Build history of the part. All positions in model axes, mm. A direction names the side the tool comes from. Coordinates: 2 decimals unless noted, no trailing zeros. Loops run counter-clockwise (first coordinate to the right, second up) from the corner with the lowest first, then second, coordinate; pieces in that order, holes last.
Item 1: Mould opens along Z. For faces 6 (the face through (9, 27, 332)), 7 (the face through (-10, 5, 211)), 8 (the face through (0, 27, 322.6)), 9 (the face through (0, 24, 341.6)) say: released by +Z, released by -Z, zero draft, split by the parting line, or undercut.
Item 2: Drill centre lines: line 1 along Z through (x, y) = (1.5, 24.5); line 2 along X through (y, z) = (-6, 237). Where is each one in solid material? Low to high.
Item 3: Cut at D-D (z = 279). List the corners of the cut face in (x, y).
Item 4: Cut at C-C (y = 2). List the corners of the cut face in (x, z), and give its area (3 significant figures).
Item 5: Cut at A-A (y = 38). List the corners of the cut face in (x, z).
Item 6: Cut at B-B (x = -5.25). List the corners of the cut face in (y, z), and give its area (3 significant figures).
Item 7: 3-axis set-ups, long thin cutter, end or side, ignore diameter. For faces 1 (the face through (-0.8, 45, 19.6)), 2 (the face through (0, 10, 10)), 3 (the face through (9, 0, 168)), 4 (the face through (0, -10, 168)), 5 (the face through (0, 27, 20)): which of +Z, -Z, +X, -X, +Y, -Y reach the whole face in a straight line?
Item 8: Flat gauge pin, fed straight in: pin 1 (4 mm diameter, centred on x = 0.5, z = 142, fed in from +Y). Where does the tip first touch, or does it go through?
from build123d import *

# Parameters (mm, degrees)
SKETCH2_W           = 20
SKETCH2_H           = 20
SKETCH2_W_2         = 18
SKETCH2_H_2         = 18
BOSS_EXTRUDE1_DEPTH = 341.6
SKETCH3_W           = 20
SKETCH3_H           = 20
SKETCH3_W_2         = 18
SKETCH3_H_2         = 18
BOSS_EXTRUDE2_DEPTH = 35


with BuildPart() as part:
    # Sketch2 → Boss-Extrude1 (new body)
    with BuildSketch(Plane.XY):
        Rectangle(SKETCH2_W, SKETCH2_H)
        Rectangle(SKETCH2_W_2, SKETCH2_H_2, mode=Mode.SUBTRACT)
    extrude(amount=BOSS_EXTRUDE1_DEPTH)

    # Sketch3 → Boss-Extrude2 (add)
    with BuildSketch(Plane(origin=(0, 10, 0), x_dir=(1, 0, 0), z_dir=(0, 1, 0))):
        with Locations((0, -10)):
            Rectangle(SKETCH3_W, SKETCH3_H)
        with Locations((0, -10)):
            Rectangle(SKETCH3_W_2, SKETCH3_H_2, mode=Mode.SUBTRACT)
        with Locations((0, -331.6)):
            Rectangle(SKETCH3_W, SKETCH3_H)
        with Locations((0, -331.6)):
            Rectangle(SKETCH3_W_2, SKETCH3_H_2, mode=Mode.SUBTRACT)
    extrude(amount=BOSS_EXTRUDE2_DEPTH)


solid = part.part
Filled sheet:
1. face 6: undercut
1. face 7: zero draft
1. face 8: undercut
1. face 9: released by +Z
2. line 1: z = 0 to 1, 19 to 20, 321.6 to 322.6, 340.6 to 341.6
2. line 2: x = -10 to -9, 9 to 10
3. outline: (-10, -10) - (10, -10) - (10, 10) - (-10, 10) - close; hole (-9, -9) - (9, -9) - (9, 9) - (-9, 9) - close
4. outline: (-10, 0) - (-9, 0) - (-9, 341.6) - (-10, 341.6) - close; (9, 0) - (10, 0) - (10, 341.6) - (9, 341.6) - close
4. area: 683 mm2
5. outline: (-10, 0) - (10, 0) - (10, 20) - (-10, 20) - close; (-10, 321.6) - (10, 321.6) - (10, 341.6) - (-10, 341.6) - close; hole (-9, 1) - (9, 1) - (9, 19) - (-9, 19) - close; hole (-9, 322.6) - (9, 322.6) - (9, 340.6) - (-9, 340.6) - close
6. outline: (-10, 0) - (-9, 0) - (-9, 341.6) - (-10, 341.6) - close; (9, 0) - (45, 0) - (45, 1) - (10, 1) - (10, 19) - (45, 19) - (45, 20) - (10, 20) - (10, 321.6) - (45, 321.6) - (45, 322.6) - (10, 322.6) - (10, 340.6) - (45, 340.6) - (45, 341.6) - (9, 341.6) - close
6. area: 823 mm2
7. face 1: +Z, -Z, +X, -X, +Y
7. face 2: +Y
7. face 3: +Z, -Z
7. face 4: +Z, -Z, +X, -X, -Y
7. face 5: +X, -X, +Y
8. pin 1: stops at y = 10
